from build123d import *

# Parameters (mm, degrees)
EXTRUDE_1_DEPTH     = 196
SKETCH_2_W          = 1
SKETCH_2_H          = 196
CUT_EXTRUDE_1_DEPTH = 1
SKETCH1_R           = 2.25
CUT_EXTRUDE1_DEPTH  = 2


with BuildPart() as part:
    # Эскиз1 → Бобышка-Вытянуть1 (new body)
    with BuildSketch(Plane(origin=(0, 0, 0), x_dir=(1, 0, 0), z_dir=(0, 1, 0))):
        Polygon((0, 0), (0, 20), (1, 20), (1, 1), (20, 1), (20, 0), align=None)
    extrude(amount=EXTRUDE_1_DEPTH)

    # Эскиз2 → Вырез-Вытянуть1 (cut)
    with BuildSketch(Plane(origin=(20, 0, 0), x_dir=(0, 0, -1), z_dir=(1, 0, 0))):
        with Locations((0.5, 98)):
            Rectangle(SKETCH_2_W, SKETCH_2_H)
    extrude(amount=-CUT_EXTRUDE_1_DEPTH, mode=Mode.SUBTRACT)

    # Sketch1 → Cut-Extrude1 (cut, through all)
    with BuildSketch(Plane(origin=(0, 0, -1), x_dir=(-1, 0, 0), z_dir=(0, 0, -1))):
        with Locations((-11, 82)):
            Circle(SKETCH1_R)
        with Locations((-11, 114)):
            Circle(SKETCH1_R)
    extrude(amount=-CUT_EXTRUDE1_DEPTH, mode=Mode.SUBTRACT)


solid = part.part
Design review of the part built by this model. Coordinates are the model's own, in mm. A direction names the side the tool comes from. Round coordinates to 2 decimals unless told otherwise and drop trailing zeros. Loops run counter-clockwise (first coordinate to the right, second up) from the corner with the lowest first, then second, coordinate; pieces in that order, holes last. Notation, with made-up numbers: (67, 34.5) -> (118, 34.5) arc R21 ccw to (118, 44.5) -> close; hole circle Ø1 at (-32.5, -0.75). An arc over 180 degrees is marked (long way). Use one line per item in the form item = value. Start each with the question number.
Q1. We need section D-D on z = -15.5. Give the boundary of the cut face in (x, y).
Q2. We need section C-C on y = 152.5. Give the boundary of the cut face in (x, z).
Q3. Machinability: for faces 4 (the face through (11.488, 79.804, -0.507)), 5 (the face through (1, 97, -11)), which of the approach directions +Z, -Z, +X, -X, +Y, -Y give a long, thin tool a straight path to every point of the face, cutting with its end or side? Answer none if there is none.
Q4. We need section B-B on x = 11. Give the boundary of the cut face in (y, z), then the cut area to 3 significant figures.
Q5. We need section A-A on y = 114. Give the boundary of the cut face in (x, z).
Q6. Wall thickness on line 1 along Y through (x, z) = (11, -0.4); line 2 along X through (y, z) = (41.5, -10.25); line 3 along Z through (x, y) = (13, 133.5): over which ranges is each line inside the solid? List them lowest first. Write a range as [from, to].
Q7. For pin 1 Ø3 at (x, y) = (16.5, 164) entering from +Z; pin 2 Ø9.5 at (y, z) = (111, -12) entering from +X; pin 3 Ø4 at (x, y) = (11, 82) entering from +Z; pin 4 Ø5.5 at (x, y) = (6, 109.5) entering from -Z, all flat-tipped, find the tip position at first contact; note any pin that passes through.
Q8. Draft analysis for pull direction Y (two halves, no side actions). For faces 1 (the face through (11.488, 111.804, -0.507)), 2 (the face through (10, 97, -1)), 3 (the face through (0.4, 196, -5.6)), state which applies: +Y half, -Y half, draft (parallel to the pull), parting line (faces both ways), or undercut.
Calculated:
q1.outline = (0, 0) -> (1, 0) -> (1, 196) -> (0, 196) -> close
q2.outline = (0, -20) -> (1, -20) -> (1, -1) -> (19, -1) -> (19, 0) -> (0, 0) -> close
q3.face_4 = +Z, -Z
q3.face_5 = -Z, +X, +Y, -Y
q4.outline = (0, -1) -> (79.75, -1) -> (79.75, 0) -> (0, 0) -> close; (84.25, -1) -> (111.75, -1) -> (111.75, 0) -> (84.25, 0) -> close; (116.25, -1) -> (196, -1) -> (196, 0) -> (116.25, 0) -> close
q4.area = 187 mm²
q5.outline = (0, -20) -> (1, -20) -> (1, -1) -> (8.75, -1) -> (8.75, 0) -> (0, 0) -> close; (13.25, -1) -> (19, -1) -> (19, 0) -> (13.25, 0) -> close
q6.line_1 = [0, 79.75], [84.25, 111.75], [116.25, 196]
q6.line_2 = [0, 1]
q6.line_3 = [-1, 0]
q7.pin_1 = 0
q7.pin_2 = 1
q7.pin_3 = through
q7.pin_4 = -1
q8.face_1 = undercut
q8.face_2 = draft
q8.face_3 = +Y half
